Build history of the part. All positions in model axes, mm. Face numbers are marked on the shaded views. Give positions to 0.01 mm unless a question says otherwise; leave off trailing zeros. Order: outer loops, then holes, each group sorted by start corner. A loop starts at its lowest first (then second) coordinate and runs counter-clockwise, first axis right, second up. Notation, with made-up numbers: (-19.5, -12.75) - (34.5, -12.75) arc R25 ccw to (34.5, 9.25) - close; hole circle Ø7 at (75.25, -25). An arc over 180 degrees is marked (long way). Use a Markdown table: item, result. Add a question column.
(1) Flat gauge pins, fed straight in: pin 1 (3 mm diameter, centred on x = -1, y = 1.5, fed in from +Z); pin 2 (3 mm diameter, centred on y = -1, z = 11, fed in from -X). Where does each tip first touch, or does it go through?
(2) Slice it at B-B (z = 11). Write the cut outline in (x, y).
(3) Slice it at A-A (x = 0). Write the cut outline in (y, z), then the cut area to 3 significant figures.
(4) Mould opens along X. For the marked faces 1, 2 and 3 say: +X half, -X half, draft (parallel to the pull), parting line (faces both ways), or undercut.
(5) Slice it at C-C (y = -1.25). Write the cut outline in (x, z).
(6) Slice it at D-D (x = -3.5). Write the cut outline in (y, z).
(7) Wall check: line 1 (Y direction, x = 0, z = 20); line 2 (X direction, y = -1.25, z = 18.5); line 3 (X direction, y = -1, z = 19). Give the ranges that are in metal, low to high.
Autodesk Inventor part; units mm, degrees
ref_plane "YZ Plane" through (0, 0, 0) normal (1, 0, 0) x (0, 1, 0)
ref_plane "XZ Plane" through (0, 0, 0) normal (0, 1, 0) x (-1, 0, 0)
ref_plane "XY Plane" through (0, 0, 0) normal (0, 0, 1) x (1, 0, 0)
sketch "Base" plane through (0, 0, 0) normal (0, 0, 1) x (1, 0, 0)
  circle A0 centre (0, 0) radius 2.5 construction
  circle A1 centre (0, 0) radius 4 construction
  line L0 (2, 3.4641) -> (4, 0)
  line L1 (4, 0) -> (2, -3.4641)
  line L2 (2, -3.4641) -> (-2, -3.4641)
  line L3 (-2, -3.4641) -> (-4, 0)
  line L4 (-4, 0) -> (-2, 3.4641)
  line L5 (-2, 3.4641) -> (2, 3.4641)
  line L6 (-5.6, 0) -> (5.6, 0)
  dimension "d1" = 8
  dimension "d0" = 5
extrude "BaseFeature" add sketch "Base" along normal blind 32
sketch "MountHole" plane through (0, 0, 32) normal (0, 0, 1) x (1, 0, 0)
  point P0 (0, 0)
hole "MountHoleFeature" at (0, 0, 32) direction (0, 0, -1) diameter 4.134 end through all
properties part number "M5-Standoff-32mm"
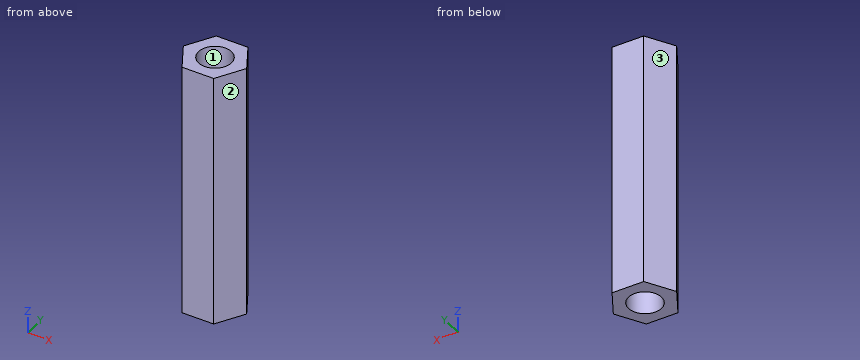
Solution:
| question | item | result |
|---|---|---|
| 1 | pin 1 | z = 32 |
| 1 | pin 2 | x = -4 |
| 2 | outline | (-4, 0) - (-2, -3.46) - (2, -3.46) - (4, 0) - (2, 3.46) - (-2, 3.46) - close; hole circle Ø4.13 at (0, 0) |
| 3 | outline | (-3.46, 0) - (-2.07, 0) - (-2.07, 32) - (-3.46, 32) - close; (2.07, 0) - (3.46, 0) - (3.46, 32) - (2.07, 32) - close |
| 3 | area | 89.4 mm2 |
| 4 | face 1 | undercut |
| 4 | face 2 | +X half |
| 4 | face 3 | -X half |
| 5 | outline | (-3.28, 0) - (-1.65, 0) - (-1.65, 32) - (-3.28, 32) - close; (1.65, 0) - (3.28, 0) - (3.28, 32) - (1.65, 32) - close |
| 6 | outline | (-0.87, 0) - (0.87, 0) - (0.87, 32) - (-0.87, 32) - close |
| 7 | line 1 | -3.46 to -2.07, 2.07 to 3.46 |
| 7 | line 2 | -3.28 to -1.65, 1.65 to 3.28 |
| 7 | line 3 | -3.42 to -1.81, 1.81 to 3.42 |
